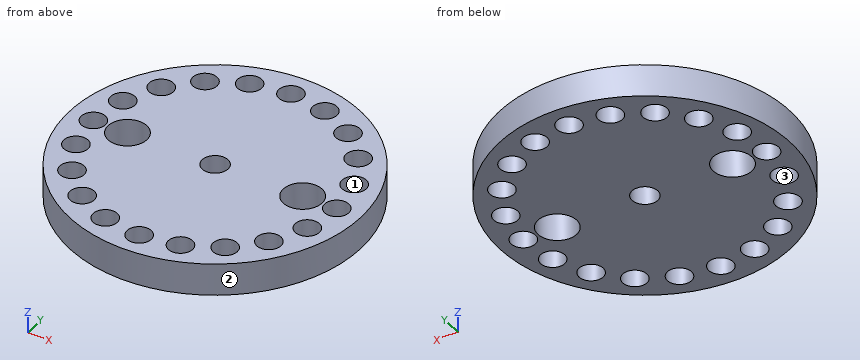
from build123d import *

# Parameters (mm, degrees)
SKETCH1_R           = 45
SKETCH1_R_2         = 3.75
BOSS_EXTRUDE1_DEPTH = 10
SKETCH2_R           = 6
CUT_EXTRUDE1_DEPTH  = 10
SKETCH3_R           = 4
CUT_EXTRUDE2_DEPTH  = 13


with BuildPart() as part:
    # Sketch1 → Boss-Extrude1 (new body)
    with BuildSketch(Plane.XY):
        Circle(SKETCH1_R)
        with Locations((0, 37.5)):
            Circle(SKETCH1_R_2, mode=Mode.SUBTRACT)
        with Locations((11.588137289, 35.664619361)):
            Circle(SKETCH1_R_2, mode=Mode.SUBTRACT)
        with Locations((22.041946961, 30.338137289)):
            Circle(SKETCH1_R_2, mode=Mode.SUBTRACT)
        with Locations((30.338137289, 22.041946961)):
            Circle(SKETCH1_R_2, mode=Mode.SUBTRACT)
        with Locations((35.664619361, 11.588137289)):
            Circle(SKETCH1_R_2, mode=Mode.SUBTRACT)
        with Locations((37.5, 0)):
            Circle(SKETCH1_R_2, mode=Mode.SUBTRACT)
        with Locations((35.664619361, -11.588137289)):
            Circle(SKETCH1_R_2, mode=Mode.SUBTRACT)
        with Locations((30.338137289, -22.041946961)):
            Circle(SKETCH1_R_2, mode=Mode.SUBTRACT)
        with Locations((22.041946961, -30.338137289)):
            Circle(SKETCH1_R_2, mode=Mode.SUBTRACT)
        with Locations((11.588137289, -35.664619361)):
            Circle(SKETCH1_R_2, mode=Mode.SUBTRACT)
        with Locations((0, -37.5)):
            Circle(SKETCH1_R_2, mode=Mode.SUBTRACT)
        with Locations((-11.588137289, -35.664619361)):
            Circle(SKETCH1_R_2, mode=Mode.SUBTRACT)
        with Locations((-22.041946961, -30.338137289)):
            Circle(SKETCH1_R_2, mode=Mode.SUBTRACT)
        with Locations((-30.338137289, -22.041946961)):
            Circle(SKETCH1_R_2, mode=Mode.SUBTRACT)
        with Locations((-35.664619361, -11.588137289)):
            Circle(SKETCH1_R_2, mode=Mode.SUBTRACT)
        with Locations((-37.5, 0)):
            Circle(SKETCH1_R_2, mode=Mode.SUBTRACT)
        with Locations((-35.664619361, 11.588137289)):
            Circle(SKETCH1_R_2, mode=Mode.SUBTRACT)
        with Locations((-30.338137289, 22.041946961)):
            Circle(SKETCH1_R_2, mode=Mode.SUBTRACT)
        with Locations((-22.041946961, 30.338137289)):
            Circle(SKETCH1_R_2, mode=Mode.SUBTRACT)
        with Locations((-11.588137289, 35.664619361)):
            Circle(SKETCH1_R_2, mode=Mode.SUBTRACT)
    extrude(amount=BOSS_EXTRUDE1_DEPTH)

    # Sketch2 → Cut-Extrude1 (cut)
    with BuildSketch(Plane(origin=(0, 0, 0), x_dir=(-1, 0, 0), z_dir=(0, 0, -1))):
        with Locations((27, 0)):
            Circle(SKETCH2_R)
        with Locations(Location((-27, 0, 0), (0, 0, 180))):
            Circle(SKETCH2_R)
    extrude(amount=-CUT_EXTRUDE1_DEPTH, mode=Mode.SUBTRACT)

    # Sketch3 → Cut-Extrude2 (cut)
    with BuildSketch(Plane(origin=(0, 0, 0), x_dir=(-1, 0, 0), z_dir=(0, 0, -1))):
        Circle(SKETCH3_R)
    extrude(amount=-CUT_EXTRUDE2_DEPTH, mode=Mode.SUBTRACT)


solid = part.part
Part model, mm, in its own coordinate system. Face numbers are marked on the shaded views. Give positions to 0.01 mm unless a question says otherwise; leave off trailing zeros. Write each loop counter-clockwise with the first axis right and the second up, starting at its lowest first coordinate (ties: lowest second). Pieces come first, ordered by that corner, then holes.
1) Probe L1, parallel to Y at x = 0, z = 6.75; L2, parallel to Y at x = -35, z = 6.75; L3, parallel to X at y = -14.5, z = 5.25. List the from-to ranges inside material, lowest first.
Resolved:
L1: y = -45 to -41.25, -33.75 to -4, 4 to 33.75, 41.25 to 45
L2: y = -28.28 to -15.28, -7.9 to -2.8, 2.8 to 7.9, 15.28 to 28.28
L3: x = -42.6 to -38.03, -33.3 to 33.3, 38.03 to 42.6
2) Cut at D-D on x = -14. Write the cut outline in (y, z).
Resolved:
outline: (-42.77, 0) - (-38.54, 0) - (-38.54, 10) - (-42.77, 10) - close; (-32.79, 0) - (32.79, 0) - (32.79, 10) - (-32.79, 10) - close; (38.54, 0) - (42.77, 0) - (42.77, 10) - (38.54, 10) - close
3) Pin check, flat tips, straight feed: pin 1 (9.5 mm diameter, centred on x = 27, y = 0, fed in from -Z); pin 2 (1 mm diameter, centred on x = 19, z = 4.5, fed in from -Y); pin 3 (4 mm diameter, centred on y = 33, z = 4.5, fed in from +X); pin 4 (2 mm diameter, centred on x = 29, z = 9, fed in from -Y). Stop position of each tip, or through.
Resolved:
pin 1: passes through
pin 2: stops at y = -41.02
pin 3: stops at x = 32.62
pin 4: stops at y = -35.23
4) Cut at A-A on y = 0. Write the cut outline in (x, z), then the cut area to 3 significant figures.
Resolved:
outline: (-45, 0) - (-41.25, 0) - (-41.25, 10) - (-45, 10) - close; (-33.75, 0) - (-33, 0) - (-33, 10) - (-33.75, 10) - close; (-21, 0) - (-4, 0) - (-4, 10) - (-21, 10) - close; (4, 0) - (21, 0) - (21, 10) - (4, 10) - close; (33, 0) - (33.75, 0) - (33.75, 10) - (33, 10) - close; (41.25, 0) - (45, 0) - (45, 10) - (41.25, 10) - close
area: 430 mm2
5) Cut at C-C on y = 37.5. Write the cut outline in (x, z), then the cut area to 3 significant figures.
Resolved:
outline: (-24.87, 0) - (-14.86, 0) - (-14.86, 10) - (-24.87, 10) - close; (-8.32, 0) - (-3.75, 0) - (-3.75, 10) - (-8.32, 10) - close; (3.75, 0) - (8.32, 0) - (8.32, 10) - (3.75, 10) - close; (14.86, 0) - (24.87, 0) - (24.87, 10) - (14.86, 10) - close
area: 292 mm2
6) Cut at B-B on x = 0. Write the cut outline in (y, z), then the cut area to 3 significant figures.
Resolved:
outline: (-45, 0) - (-41.25, 0) - (-41.25, 10) - (-45, 10) - close; (-33.75, 0) - (-4, 0) - (-4, 10) - (-33.75, 10) - close; (4, 0) - (33.75, 0) - (33.75, 10) - (4, 10) - close; (41.25, 0) - (45, 0) - (45, 10) - (41.25, 10) - close
area: 670 mm2
7) Two-plate mould, pull along X, no slides. Class the marked faces 1, 2 and 3: released by +X, released by -X, zero draft, split by the parting line, or undercut.
Resolved:
face 1: undercut
face 2: split by the parting line
face 3: undercut
